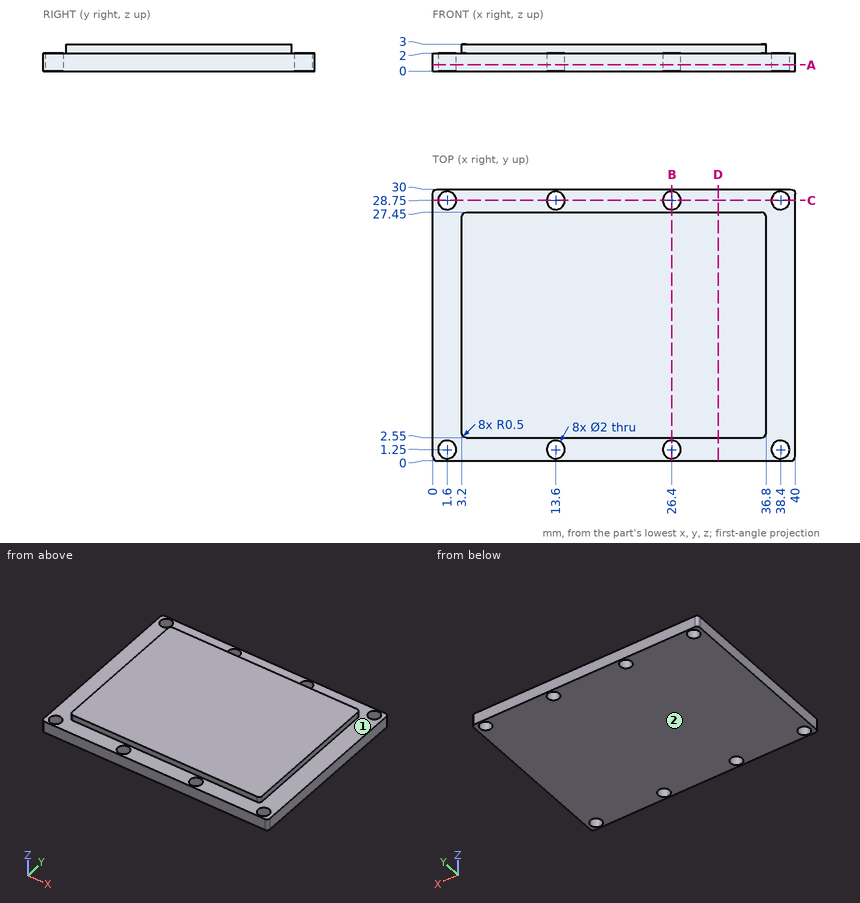
Design review of the part shown in the three views and the two pictorial views. Dimensions are in mm from the part's minimum x, y and z. A direction names the side the tool comes from. Give positions to 0.01 mm unless a question says otherwise; leave off trailing zeros. Loops run counter-clockwise (first coordinate to the right, second up) from the corner with the lowest first, then second, coordinate; pieces in that order, holes last. Notation, with made-up numbers: M 75,-16.75 L 109,-16.75 A28 cw 109,1.25 Z; hole C 83,71 d5. An arc over 180 degrees is marked long. Answer as a JSON object with one key per item and string values. Group by question number.
Q1. For probe 1 along Y at (x, z) = (13.6, 1.1); probe 2 along X at (y, z) = (28.5, 0.9); probe 3 along Y at (x, z) = (27, 1.3), list the stretches that pass through material, from the lowest coordinate up. Write a range as [from, to].
Q2. Tool access review of the marked faces 1 and 2: name each direction out of +Z, -Z, +X, -X, +Y, -Y from which nothing blocks a thin tool from reaching the whole face with its end or side.
Q3. Add section D-D on x = 31.5. Give the boundary of the cut face in (y, z).
Q4. Add section B-B on x = 26.4. Give the boundary of the cut face in (y, z), and give its area (3 significant figures).
Q5. Add section C-C on y = 28.75. Give the boundary of the cut face in (x, z), and give its area (3 significant figures).
Q6. Add section A-A on z = 0.7. Give the number of separate pieces and of enclosed holes in the cut face, and give its area (3 significant figures).
Q7. Insertion check: P1, Ø0.8, axis at x = 27.5, z = 2.5, coming from the -Y side; P2, Ø1.8, axis at x = 1.6, y = 1.25, coming from the -Z side; P3, Ø1, axis at x = 18, z = 1, coming from the -Y side; P4, Ø2.5, axis at x = 1.6, y = 28.75, coming from the +Z side. Each pin has a flat end and moves straight along its axis. Give the tip position at first contact, or say it passes through.
Checked values:
{
 "1": {"probe 1": "[0, 0.25], [2.25, 27.75], [29.75, 30]", "probe 2": "[0, 0.63], [2.57, 12.63], [14.57, 25.43], [27.37, 37.43], [39.37, 40]", "probe 3": "[0, 0.45], [2.05, 27.95], [29.55, 30]"},
 "2": {"face 1": "+Z", "face 2": "-Z, +X, -X, +Y, -Y"},
 "3": {"outline": "M 0,0 L 30,0 L 30,2 L 27.45,2 L 27.45,3 L 2.55,3 L 2.55,2 L 0,2 Z"},
 "4": {"outline": "M 0,0 L 0.25,0 L 0.25,2 L 0,2 Z; M 2.25,0 L 27.75,0 L 27.75,2 L 27.45,2 L 27.45,3 L 2.55,3 L 2.55,2 L 2.25,2 Z; M 29.75,0 L 30,0 L 30,2 L 29.75,2 Z", "area": "76.9 mm²"},
 "5": {"outline": "M 0,0 L 0.6,0 L 0.6,2 L 0,2 Z; M 2.6,0 L 12.6,0 L 12.6,2 L 2.6,2 Z; M 14.6,0 L 25.4,0 L 25.4,2 L 14.6,2 Z; M 27.4,0 L 37.4,0 L 37.4,2 L 27.4,2 Z; M 39.4,0 L 40,0 L 40,2 L 39.4,2 Z", "area": "64.0 mm²"},
 "6": {"separate pieces": "1", "enclosed holes": "8", "area": "1,170 mm²"},
 "7": {"P1": "y = 2.55", "P2": "through", "P3": "y = 0", "P4": "z = 2"}
}
